from build123d import *

# Parameters (mm, degrees)
BOSS_EXTRUDE1_DEPTH            = 215.9
CUT_EXTRUDE1_DEPTH             = 218.110576665
F_5_16_0_3125_DIAMETER_HOLE1_D = 7.9375


with BuildPart() as part:
    # Sketch1 → Boss-Extrude1 (new, symmetric)
    with BuildSketch(Plane.XY):
        Polygon((-19.05, -6.35), (-6.35, 6.35), (19.05, 6.35), (19.05, -6.35), align=None)
    extrude(amount=BOSS_EXTRUDE1_DEPTH, both=True)

    # Sketch2 → Cut-Extrude1 (cut, through all)
    with BuildSketch(Plane(origin=(0, 6.35, 0), x_dir=(1, 0, 0), z_dir=(0, 1, 0))):
        Polygon((19.05, 215.9), (-19.05, 215.9), (19.05, 177.8), align=None)
    extrude(amount=-CUT_EXTRUDE1_DEPTH, mode=Mode.SUBTRACT)

    # 5/16 (0.3125) Diameter Hole1 (through all)
    with Locations(Plane(origin=(0, 6.35, 0), x_dir=(1, 0, 0), z_dir=(0, 1, 0))):
        with Locations((7.9375, 168.275), (7.9375, 0), (7.9375, -187.325)):
            Hole(F_5_16_0_3125_DIAMETER_HOLE1_D / 2)


solid = part.part
Verification items for the finished model (mm, model axes). Round coordinates to 2 decimals unless told otherwise and drop trailing zeros. Write each loop counter-clockwise with the first axis right and the second up, starting at its lowest first coordinate (ties: lowest second). Pieces come first, ordered by that corner, then holes.
(1) Material ranges on line 1 (Z direction, x = 6, y = 1); line 2 (Z direction, x = 8.5, y = -1.75); line 3 (Y direction, x = -12, z = -115.5), recorded low to high.
Returned:
line 1: z = -190.85 to -171.74, -164.81 to -3.46, 3.46 to 183.86, 190.79 to 215.9
line 2: z = -188.35 to -172.2, -164.35 to -3.93, 3.93 to 183.4, 191.25 to 215.9
line 3: y = -6.35 to 0.7
(2) Depth check by flat-ended pin: pin 1 Ø6 at (x, y) = (9, 0) entering from -Z; pin 2 Ø1.5 at (x, y) = (6, 3.5) entering from -Z; pin 3 Ø4 at (x, y) = (12.5, 3) entering from -Z. Enter the tip coordinate at first touch or a pass-through.
Returned:
pin 1: stops at z = -190.85
pin 2: stops at z = -191.6
pin 3: stops at z = -186.35
(3) Section check C-C (x = -1). Enter the section's corners in (y, z), plus the area to 3 significant figures.
Returned:
outline: (-6.35, -197.85) - (6.35, -197.85) - (6.35, 215.9) - (-6.35, 215.9) - close
area: 5,250 mm2
(4) Section check D-D (z = 80). Enter the section's corners in (x, y), plus the area to 3 significant figures.
Returned:
outline: (-19.05, -6.35) - (19.05, -6.35) - (19.05, 6.35) - (-6.35, 6.35) - close
area: 403 mm2
(5) Section check A-A (z = 0). Enter the section's corners in (x, y).
Returned:
outline: (-19.05, -6.35) - (3.97, -6.35) - (3.97, 6.35) - (-6.35, 6.35) - close; (11.91, -6.35) - (19.05, -6.35) - (19.05, 6.35) - (11.91, 6.35) - close
(6) Mould release check, pull along Z, two halves, no side actions. Record for faces 1 (the cylindrical face through (11.087, -0.089, -165.86)), 2 (the flat face through (19.05, 0, 22)), 3 (the cylindrical face through (8.8, -0.1, 191.2)), 4 (the flat face through (3.97, 0.09, -192.88)): pulls with the +Z half, pulls with the -Z half, needs draft (parallel to the pull), parting line crosses it, or undercut.
Returned:
face 1: undercut
face 2: needs draft
face 3: undercut
face 4: pulls with the -Z half
(7) Section check B-B (y = 2). Give the number of separate pieces and of enclosed holes in the cut face, plus the area to 3 significant figures.
Returned:
separate pieces: 1
enclosed holes: 3
area: 12,000 mm2
